```python
from build123d import *

# Parameters (mm, degrees)
SKETCH1_W           = 75.9
SKETCH1_H           = 100
BOSS_EXTRUDE1_DEPTH = 20
SKETCH2_R           = 2.5
CUT_EXTRUDE1_DEPTH  = 85.734786653
SKETCH3_W           = 27.95
SKETCH3_H           = 100
CUT_EXTRUDE2_DEPTH  = 85.734786653
SKETCH4_W           = 7
SKETCH4_H           = 25
CUT_EXTRUDE3_DEPTH  = 41
SKETCH5_R           = 2
CUT_EXTRUDE4_DEPTH  = 69.0951966
SKETCH6_R           = 2
CUT_EXTRUDE5_DEPTH  = 64.589352813


with BuildPart() as part:
    # Sketch1 → Boss-Extrude1 (new body)
    with BuildSketch(Plane.XY):
        with Locations((-21.517455621, 6.952662722)):
            Rectangle(SKETCH1_W, SKETCH1_H)
    extrude(amount=BOSS_EXTRUDE1_DEPTH)

    # Sketch2 → Cut-Extrude1 (cut, through all)
    with BuildSketch(Plane.XY.offset(20)):
        with Locations((-21.517455621, 28.952662722)):
            Circle(SKETCH2_R)
    extrude(amount=-CUT_EXTRUDE1_DEPTH, mode=Mode.SUBTRACT)

    # Sketch3 → Cut-Extrude2 (cut, through all)
    with BuildSketch(Plane.XY.offset(20)):
        with Locations((-45.492455621, 6.952662722)):
            Rectangle(SKETCH3_W, SKETCH3_H)
        with Locations((2.457544379, 6.952662722)):
            Rectangle(SKETCH3_W, SKETCH3_H)
    extrude(amount=-CUT_EXTRUDE2_DEPTH, mode=Mode.SUBTRACT)

    # Sketch4 → Cut-Extrude3 (cut)
    with BuildSketch(Plane(origin=(-11.517455621, 0, 0), x_dir=(0, 0, -1), z_dir=(1, 0, 0))):
        with Locations((-11.75, 29.452662722)):
            Rectangle(SKETCH4_W, SKETCH4_H)
    extrude(amount=-CUT_EXTRUDE3_DEPTH, mode=Mode.SUBTRACT)

    # Sketch5 → Cut-Extrude4 (cut, through all)
    with BuildSketch(Plane.XY.offset(20)):
        with Locations((-21.517455621, -3.047337278)):
            Circle(SKETCH5_R)
        with Locations((-21.517455621, -23.047337278)):
            Circle(SKETCH5_R)
    extrude(amount=-CUT_EXTRUDE4_DEPTH, mode=Mode.SUBTRACT)

    # Sketch6 → Cut-Extrude5 (cut, through all)
    with BuildSketch(Plane(origin=(-11.517455621, 0, 0), x_dir=(0, 0, -1), z_dir=(1, 0, 0))):
        with Locations(Location((-10, -13.047337278, 0), (0, 0, 90))):
            Circle(SKETCH6_R)
        with Locations(Location((-10, -28.047337278, 0), (0, 0, 90))):
            Circle(SKETCH6_R)
    extrude(amount=-CUT_EXTRUDE5_DEPTH, mode=Mode.SUBTRACT)


solid = part.part
```
Geometry check sheet. Reference: the model listing, model coordinates, mm. A direction names the side the tool comes from. Coordinates: 2 decimals unless noted, no trailing zeros. Order: outer loops, then holes, each group sorted by start corner. A loop starts at its lowest first (then second) coordinate and runs counter-clockwise, first axis right, second up. Notation, with made-up numbers: (24.5, 39.25) - (49.5, 39.25) arc R18 ccw to (49.5, 52.25) - close; hole circle Ø4 at (-16, 74). An arc over 180 degrees is marked (long way). Answer in a Markdown table with one row per item. Add a question column.
1. Section check C-C (z = 18.75). Enter the section's corners in (x, y), plus the area to 3 significant figures.
2. Draft check along Y on faces 3 (the face through (-22, 8, 20)), 4 (the face through (-22.059, 26.512, 17.658)), 5 (the face through (-22, 56.953, 10)). Enter one of: +Y half, -Y half, draft (parallel to the pull), parting line (faces both ways), or undercut.
3. Material ranges on L1, parallel to Y at x = -21.75, z = 7.25; L2, parallel to Z at x = -26.5, y = 33; L3, parallel to Y at x = -22.75, z = 2.5, recorded low to high. Write a range as [from, to].
4. Section check A-A (z = 10). Enter the section's corners in (x, y).
5. Access from +Z, -Z, +X, -X, +Y, -Y to the whole of each face (thin tool, end or side, straight path). Record for faces 1 (the face through (-21, 32, 8.25)), 2 (the face through (-19.67, -3.81, 10.14)).
6. Section check B-B (x = -14). Enter the section's corners in (y, z), plus the area to 3 significant figures.
7. Gauge pin test, flat end, axial feed: pin 1 Ø2.5 at (x, y) = (-21.52, -23.05) entering from -Z. Record the tip position at first contact, or that the pin passes through.
Data:
| question | item | result |
|---|---|---|
| 1 | outline | (-31.52, -43.05) - (-11.52, -43.05) - (-11.52, 56.95) - (-31.52, 56.95) - close; hole circle Ø5 at (-21.52, 28.95); hole circle Ø4 at (-21.52, -23.05); hole circle Ø4 at (-21.52, -3.05) |
| 1 | area | 1,960 mm² |
| 2 | face 3 | draft |
| 2 | face 4 | undercut |
| 2 | face 5 | +Y half |
| 3 | L1 | y = [-43.05, -25.03], [-21.06, -5.03], [-1.06, 26.46], [31.44, 56.95] |
| 3 | L2 | z = [0, 8.25], [15.25, 20] |
| 3 | L3 | y = [-43.05, -24.62], [-21.47, -4.62], [-1.47, 26.78], [31.13, 56.95] |
| 4 | outline | (-31.52, -43.05) - (-11.52, -43.05) - (-11.52, -30.05) - (-31.52, -30.05) - close; (-31.52, -26.05) - (-11.52, -26.05) - (-11.52, -15.05) - (-31.52, -15.05) - close; (-31.52, -11.05) - (-11.52, -11.05) - (-11.52, 16.95) - (-31.52, 16.95) - close; (-31.52, 41.95) - (-11.52, 41.95) - (-11.52, 56.95) - (-31.52, 56.95) - close; hole circle Ø4 at (-21.52, -23.05); hole circle Ø4 at (-21.52, -3.05) |
| 5 | face 1 | +X, -X |
| 5 | face 2 | +Z, -Z |
| 6 | outline | (-43.05, 0) - (56.95, 0) - (56.95, 20) - (-43.05, 20) - close; hole circle Ø4 at (-28.05, 10); hole circle Ø4 at (-13.05, 10); hole (16.95, 8.25) - (41.95, 8.25) - (41.95, 15.25) - (16.95, 15.25) - close |
| 6 | area | 1,800 mm² |
| 7 | pin 1 | passes through |
